Print and shaded views of the part. All mm, measured from the part's lowest x, y and z. A direction names the side the tool comes from. Round coordinates to 2 decimals unless told otherwise and drop trailing zeros. Write each loop counter-clockwise with the first axis right and the second up, starting at its lowest first coordinate (ties: lowest second). Pieces come first, ordered by that corner, then holes. Notation, with made-up numbers: (1, 25.25) - (17, 25.25) arc R14 ccw to (17, 49.25) - close; hole circle Ø9 at (39.25, 87). An arc over 180 degrees is marked (long way). Put each result on its own line as item: value. Start each with the question number.
Item 1: Pin check, flat tips, straight feed: pin 1 Ø1.5 at (y, z) = (16, 7) entering from +X (1 decimal); pin 2 Ø6 at (x, y) = (10.13, 12.5) entering from +Z; pin 3 Ø3 at (x, y) = (28.5, 11) entering from +Z; pin 4 Ø5 at (y, z) = (9, 12) entering from +X. Stop position of each tip, or through.
Item 2: 3-axis set-ups, long thin cutter, end or side, ignore diameter. For the marked faces 4, 5 and 6: which of +Z, -Z, +X, -X, +Y, -Y reach the whole face in a straight line?
Item 3: Cut at C-C (z = 10.25). Give the cut face in (x, y) (1 decimal).
Item 4: Mould opens along X. For the marked faces 1, 2 and 3 say: released by +X, released by -X, zero draft, split by the parting line, or undercut.
Item 5: Cut at A-A (y = 12.5). Give the cut face in (x, z), and give its area (3 significant figures).
Item 6: Cut at D-D (x = 16.5). Give the cut face in (y, z).
Item 7: Cut at B-B (y = 3). Give the cut face in (x, z), and give its area (3 significant figures).
Item 8: Drill centre lines: line 1 (Z direction, x = 58.5, y = 24); line 2 (X direction, y = 17.75, z = 2.75) (1 decimal); line 3 (Z direction, x = 41, y = 9.5) (1 decimal). Where is each one in solid material? Low to high. Write a range as from..to.
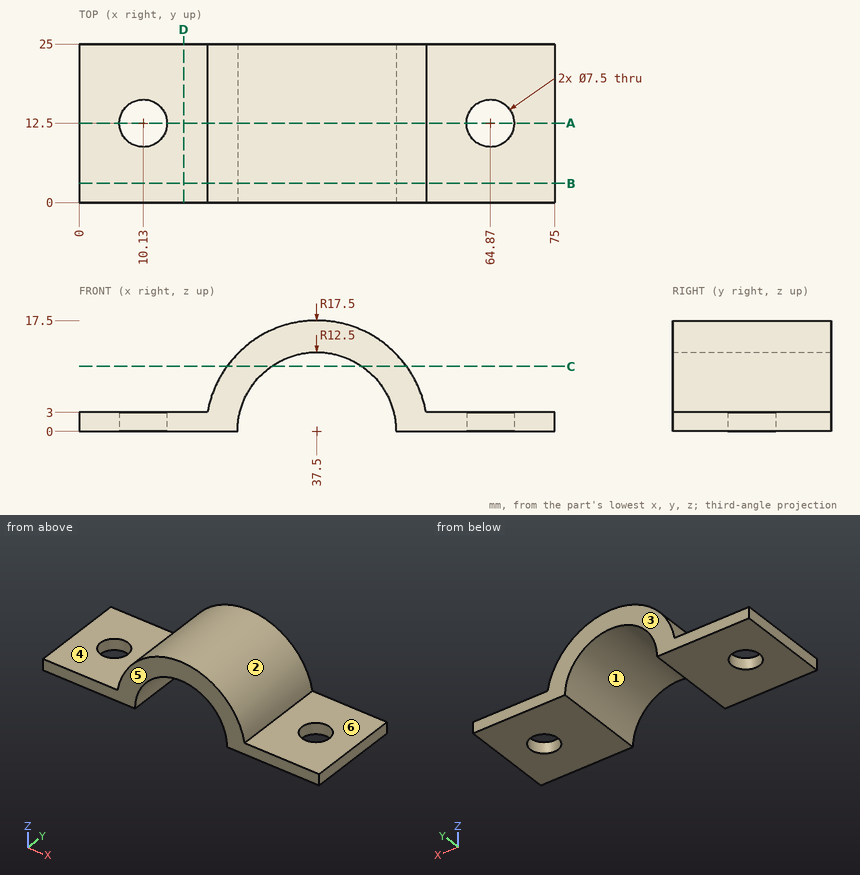
Output values:
1. pin 1: x = 53.8
1. pin 2: through
1. pin 3: z = 15.81
1. pin 4: x = 52.2
2. face 4: +Z, -X, +Y, -Y
2. face 5: +Z, -Z, +X, -X, -Y
2. face 6: +Z, +X, +Y, -Y
3. outline: (23.3, 0) - (30.3, 0) - (30.3, 25) - (23.3, 25) - close; (44.7, 0) - (51.7, 0) - (51.7, 25) - (44.7, 25) - close
4. face 1: undercut
4. face 2: split by the parting line
4. face 3: zero draft
5. outline: (0, 0) - (6.38, 0) - (6.38, 3) - (0, 3) - close; (13.88, 0) - (25, 0) arc R12.5 cw to (50, 0) - (61.12, 0) - (61.12, 3) - (54.74, 3) arc R17.5 ccw to (20.26, 3) - (13.88, 3) - close; (68.62, 0) - (75, 0) - (75, 3) - (68.62, 3) - close
5. area: 311 mm2
6. outline: (0, 0) - (25, 0) - (25, 3) - (0, 3) - close
7. outline: (0, 0) - (25, 0) arc R12.5 cw to (50, 0) - (75, 0) - (75, 3) - (54.74, 3) arc R17.5 ccw to (20.26, 3) - (0, 3) - close
7. area: 356 mm2
8. line 1: 0..3
8. line 2: 0..25.3, 49.7..75
8. line 3: 12..17.1
